```python
from build123d import *

# Parameters (mm, degrees)
BASPROSKE_W        = 12
BASPROSKE_H        = 24
TOOTHCUT_DEPTH     = 37
TEETHCUTS_COUNT    = 30
TEETHCUTS_ANGLE    = 348
BORSKE_R           = 0.4
BORE_DEPTH         = 50.0000508
SKETCH1_R          = 33.841637192
CUT_EXTRUDE1_DEPTH = 6
CUT_EXTRUDE2_DEPTH = 6


with BuildPart() as part:
    # BasProSke → Base-Revolve (revolve)
    with BuildSketch(Plane(origin=(0, 0, 0), x_dir=(1, 0, 0), z_dir=(0, 1, 0)), mode=Mode.PRIVATE) as base_revolve_sk:
        with Locations((6, 12)):
            Rectangle(BASPROSKE_W, BASPROSKE_H)
    revolve(base_revolve_sk.sketch.rotate(Axis((-10, 0, 0), (1, 0, 0)), 180), axis=Axis((-10, 0, 0), (1, 0, 0)))

    # TooCutSke → ToothCut (cut, through all)
    with BuildSketch(Plane(origin=(0, 0, 0), x_dir=(0, 0, -1), z_dir=(1, 0, 0))):
        with BuildLine():
            ThreePointArc((0.693278797, 20.612344372), (0, 20.624), (-0.693278797, 20.612344372))
            ThreePointArc((-0.693278797, 20.612344372), (-1.219042225, 22.34383125), (-2.080549663, 23.935144835))
            ThreePointArc((-2.080549663, 23.935144835), (0, 24.0254), (2.080549663, 23.935144835))
            ThreePointArc((2.080549663, 23.935144835), (1.219042225, 22.34383125), (0.693278797, 20.612344372))
        make_face()
    toothcut = extrude(amount=TOOTHCUT_DEPTH, mode=Mode.SUBTRACT)

    # TeethCuts: ToothCut ×30 about axis
    teethcuts_axis = Axis((-10, 0, 0), (1, 0, 0))
    for i in range(1, TEETHCUTS_COUNT):
        add(toothcut.rotate(teethcuts_axis, i * TEETHCUTS_ANGLE / (TEETHCUTS_COUNT - 1)), mode=Mode.SUBTRACT)

    # BorSke → Bore (cut, symmetric)
    with BuildSketch(Plane(origin=(0, 0, 0), x_dir=(0, 0, -1), z_dir=(1, 0, 0))):
        with Locations(Location((0, 0, 0), (0, 0, 180))):
            Circle(BORSKE_R)
    extrude(amount=BORE_DEPTH, both=True, mode=Mode.SUBTRACT)

    # Sketch1 → Cut-Extrude1 (cut)
    with BuildSketch(Plane.ZY):
        with Locations((-0.4, 0)):
            Circle(SKETCH1_R)
    extrude(amount=-CUT_EXTRUDE1_DEPTH, mode=Mode.SUBTRACT)

    # Sketch2 → Cut-Extrude2 (cut)
    with BuildSketch(Plane.ZY.offset(-6)):
        with BuildLine():
            ThreePointArc((4, 0), (1.732050808, 3.605551275), (-2.5, 3.122498999))
            Line((-2.5, 3.122498999), (-2.5, -3.122498999))
            ThreePointArc((-2.5, -3.122498999), (1.732050808, -3.605551275), (4, 0))
        make_face()
    extrude(amount=-CUT_EXTRUDE2_DEPTH, mode=Mode.SUBTRACT)


solid = part.part
```
Input: part model. Units: mm. Frame: model coordinates. A direction names the side the tool comes from. Give positions to 0.01 mm unless a question says otherwise; leave off trailing zeros. Write each loop counter-clockwise with the first axis right and the second up, starting at its lowest first coordinate (ties: lowest second). Pieces come first, ordered by that corner, then holes. Notation, with made-up numbers: (16.5, 53.5) - (73.5, 53.5) arc R11 ccw to (73.5, 72.5) - close; hole circle Ø4 at (74, 24). An arc over 180 degrees is marked (long way). Write item = value, one per line. Start each with the question number.
1) Cut plane B-B (y = -11.5). Return loops of the section in (x, z), and give its area (3 significant figures).
2) Pin query (flat end, axial travel): pin 1 (3 mm diameter, centred on x = 7.5, z = -15, fed in from +Y); pin 2 (2 mm diameter, centred on x = 9, y = 4.5, fed in from -Z); pin 3 (2 mm diameter, centred on x = 10.5, z = -3.5, fed in from -Y). Return the tip coordinate at first contact, or that it passes through.
3) Draft query along Z for faces 1 (the face through (8.958, -18.837, 8.397)), 2 (the face through (8.96, -8.07, -20.88)), 3 (the face through (8.96, 12.24, 18.75)). Return one class per face: pulls with the +Z half, pulls with the -Z half, needs draft (parallel to the pull), parting line crosses it, or undercut.
4) Material intervals for L1, parallel to Z at x = 8.8, y = -19.5; L2, parallel to Y at x = 11.55, z = -18.5; L3, parallel to Z at x = 11.7, y = -22, sorted ascending. Write a range as [from, to].
5) Reachability of faces 4 (the face through (8.96, 3.53, -22.06)), 5 (the face through (8.96, 20.17, -4.3)), 6 (the face through (9, -16.7, 12.1)) from +Z, -Z, +X, -X, +Y, -Y: full face, straight path, thin tool, end or side. Return the list, or none.
6) Cut plane A-A (y = 12). Return loops of the section in (x, z).
Answers follow:
q1.outline = (6, -18.12) - (12, -18.12) - (12, 18.12) - (6, 18.12) - close
q1.area = 217 mm^2
q2.pin_1 = 18.13
q2.pin_2 = -23.56
q2.pin_3 = -23.87
q3.face_1 = undercut
q3.face_2 = pulls with the -Z half
q3.face_3 = pulls with the +Z half
q4.L1 = [-12.29, -9.79], [-7.83, 7.83], [9.79, 12.29]
q4.L2 = [-14.35, -11.93], [-9.8, 9.8], [11.93, 14.35]
q4.L3 = [-7.93, -6.13], [-3.47, -1.08], [1.08, 3.47], [6.13, 7.93]
q5.face_4 = -Z, +X, -X
q5.face_5 = +X, -X, +Y
q5.face_6 = +X, -X
q6.outline = (6, -18.56) - (12, -18.56) - (12, 18.56) - (6, 18.56) - close
